Could you check a few things on this model? Use its own coordinates, in mm. A direction names the side the tool comes from. Give positions to 0.01 mm unless a question says otherwise; leave off trailing zeros. Write each loop counter-clockwise with the first axis right and the second up, starting at its lowest first coordinate (ties: lowest second). Pieces come first, ordered by that corner, then holes. Notation, with made-up numbers: (86.25, -18) -> (139.25, -18) arc R9 cw to (139.25, -7) -> close; hole circle Ø5 at (-34, 53.25). An arc over 180 degrees is marked (long way). One line per question, with ' | ' between items.
from build123d import *

# Parameters (mm, degrees)
SKETCH1_R           = 5
SKETCH1_W           = 6.6
SKETCH1_H           = 5.1
BOSS_EXTRUDE1_DEPTH = 5
SKETCH2_R           = 5
BOSS_EXTRUDE2_DEPTH = 1
SKETCH3_R           = 2.1
BOSS_EXTRUDE3_DEPTH = 8.5
SKETCH4_W           = 4.4
SKETCH4_H           = 4.4
BOSS_EXTRUDE4_DEPTH = 2


with BuildPart() as part:
    # Sketch1 → Boss-Extrude1 (new body)
    with BuildSketch(Plane(origin=(0, 0, 0), x_dir=(1, 0, 0), z_dir=(0, 1, 0))):
        Circle(SKETCH1_R)
        Rectangle(SKETCH1_W, SKETCH1_H, mode=Mode.SUBTRACT)
    extrude(amount=BOSS_EXTRUDE1_DEPTH)

    # Sketch2 → Boss-Extrude2 (add)
    with BuildSketch(Plane(origin=(0, 5, 0), x_dir=(1, 0, 0), z_dir=(0, 1, 0))):
        Circle(SKETCH2_R)
    extrude(amount=BOSS_EXTRUDE2_DEPTH)

    # Sketch3 → Boss-Extrude3 (add)
    with BuildSketch(Plane(origin=(0, 6, 0), x_dir=(1, 0, 0), z_dir=(0, 1, 0))):
        Circle(SKETCH3_R)
    extrude(amount=BOSS_EXTRUDE3_DEPTH)

    # Sketch4 → Boss-Extrude4 (add)
    with BuildSketch(Plane(origin=(0, 14.5, 0), x_dir=(1, 0, 0), z_dir=(0, 1, 0))):
        Rectangle(SKETCH4_W, SKETCH4_H)
    extrude(amount=BOSS_EXTRUDE4_DEPTH)


solid = part.part
Q1. Imagine slicing it at B-B on x = 0. Please give me the cut outline in (y, z), and give its area (3 significant figures).
Answer below:
outline: (0, -5) -> (6, -5) -> (6, -2.1) -> (14.5, -2.1) -> (14.5, -2.2) -> (16.5, -2.2) -> (16.5, 2.2) -> (14.5, 2.2) -> (14.5, 2.1) -> (6, 2.1) -> (6, 5) -> (0, 5) -> (0, 2.55) -> (5, 2.55) -> (5, -2.55) -> (0, -2.55) -> close | area: 79.0 mm^2
Q2. If we mould it in two halves opening along X, with no side actions, what happens to faces 1 (the flat face through (0, 15, 2.2)), 2 (the flat face through (0, 5, 0)), 3 (the cylindrical face through (-1.08, 2.96, 4.88))? For each: +X half, -X half, draft (parallel to the pull), parting line (faces both ways), or undercut.
Answer below:
face 1: draft | face 2: undercut | face 3: parting line
Q3. Imagine slicing it at D-D on z = -2.75. Please give me the cut outline in (x, y), and give its area (3 significant figures).
Answer below:
outline: (-4.18, 0) -> (4.18, 0) -> (4.18, 6) -> (-4.18, 6) -> close | area: 50.1 mm^2
Q4. If I drill on line 1 along Y through (x, z) = (0.75, 2); line 2 along X through (y, z) = (15.25, -2); line 3 along Y through (x, z) = (0.5, 3.5), over which ranges is the centre line in solid material (lowest first)?
Answer below:
line 1: y = 5 to 6, 14.5 to 16.5 | line 2: x = -2.2 to 2.2 | line 3: y = 0 to 6
Q5. On a 3-axis mill with a long thin cutter (end or side, diameter ignored), from which of +Z, -Z, +X, -X, +Y, -Y can I reach the whole of each face in a straight line? I mean faces 4 (the flat face through (1, 6, 2.2)), 5 (the flat face through (-2.2, 15, 0)), 6 (the flat face through (2.2, 15, 0)), 7 (the flat face through (0, 15, -2.2)). Say none if no direction works.
Answer below:
face 4: none | face 5: +Z, -Z, -X, +Y | face 6: +Z, -Z, +X, +Y | face 7: -Z, +X, -X, +Y
Q6. Imagine slicing it at C-C on x = 4. Please give me the cut outline in (y, z).
Answer below:
outline: (0, -3) -> (6, -3) -> (6, 3) -> (0, 3) -> close
Q7. Will these pins go through, and if not, where does the flat tip stop? pin 1 (1.5 mm diameter, centred on x = 0.5, y = 3.5, fed in from -Z); pin 2 (2 mm diameter, centred on x = -1, y = 12, fed in from +Z); pin 3 (1 mm diameter, centred on y = 15.5, z = 0, fed in from -X); pin 4 (2.5 mm diameter, centred on x = -1.5, z = -0.5, fed in from -Y).
Answer below:
pin 1: stops at z = -5 | pin 2: stops at z = 2.1 | pin 3: stops at x = -2.2 | pin 4: stops at y = 5
Q8. Imagine slicing it at A-A on z = 0. Please give me the cut outline in (x, y), and give its area (3 significant figures).
Answer below:
outline: (-5, 0) -> (-3.3, 0) -> (-3.3, 5) -> (3.3, 5) -> (3.3, 0) -> (5, 0) -> (5, 6) -> (2.1, 6) -> (2.1, 14.5) -> (2.2, 14.5) -> (2.2, 16.5) -> (-2.2, 16.5) -> (-2.2, 14.5) -> (-2.1, 14.5) -> (-2.1, 6) -> (-5, 6) -> close | area: 71.5 mm^2
